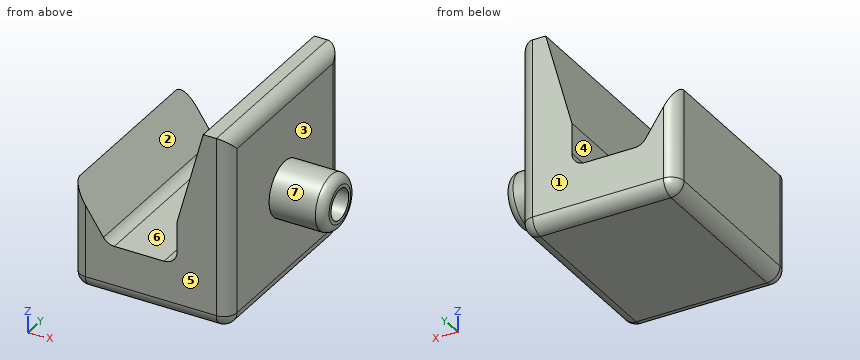
```python
from build123d import *

# Parameters (mm, degrees)
F1_DEPTH      = 11
F1_DEPTH_BACK = 11
F2_R          = 3.135192
F2_R_2        = 1.742831
F3_DEPTH      = 6.3
F4_R          = 1.5
F5_R          = 1
F3_FACE_R     = 1.742831
F6_DEPTH      = 1.5


with BuildPart() as f1:
    # F0 (on Front) → F1 (new body, two sides)
    with BuildSketch(Plane.XZ) as f1_sk:
        Polygon((-3, -11), (3, -11), (3, -3.201166), (3, 0), (3, 3.152842), (3, 11), (0, 11), (-3, 0), (-3, -5), (-11.005839, -5), (-15, 1), (-15, -5), (-15, -11), align=None)
    extrude(amount=F1_DEPTH)
    extrude(f1_sk.sketch, amount=-F1_DEPTH_BACK)

    # F2 (on face) → F3 (join)
    with BuildSketch(Plane.YZ.offset(3)):
        Circle(F2_R)
        Circle(F2_R_2, mode=Mode.SUBTRACT)
    extrude(amount=F3_DEPTH)

    # F4
    f4_edges = [f1.edges().sort_by_distance(p)[0] for p in [
        (3, -11, 0),
        (-6, -11, -11),
        (-15, -11, -5),
        (3, 0, 11),
        (3, 11, 0),
        (3, 0, -11),
        (-15, 11, -5),
        (-15, 0, -11),
        (-6, 11, -11),
        (-3, 0, -5),
        (-11.005839, 0, -5),
    ]]
    fillet(f4_edges, radius=F4_R)

    # F5
    f5_edges = [f1.edges().sort_by_distance(p)[0] for p in [
        (9.3, -3.135192, 0),
    ]]
    fillet(f5_edges, radius=F5_R)

    # F3_face (on face) → F6 (join)
    with BuildSketch(Plane.YZ.offset(3)):
        Circle(F3_FACE_R)
    extrude(amount=-F6_DEPTH)


solid = f1.part
```
Read the model definition and answer for the solid it produces. Units are mm, in the model's axes. Face numbers are marked on the shaded views. A direction names the side the tool comes from. Give positions to 0.01 mm unless a question says otherwise; leave off trailing zeros. Write each loop counter-clockwise with the first axis right and the second up, starting at its lowest first coordinate (ties: lowest second). Pieces come first, ordered by that corner, then holes. Notation, with made-up numbers: (63, 73) -> (114, 73) arc R23 ccw to (114, 102) -> close; hole circle Ø2 at (1.25, 69.25). An arc over 180 degrees is marked (long way). Answer as a JSON object with one key per item and string values.
1) Section D-D on x = 6 is taken. Write down the section's boundary in (y, z).
Findings below:
{"outline": "circle Ø6.27 at (0, 0); hole circle Ø3.49 at (0, 0)"}
2) A tool of negligible diameter and unlimited length cuts with its end or side. For the marked faces 5, 6 and 7, from which of +Z, -Z, +X, -X, +Y, -Y can it reach the whole face along a straight path? Write none if from no direction.
Findings below:
{"face 5": "+Z, -Z, +X, -X, -Y", "face 6": "+Z, +Y, -Y", "face 7": "+X"}
3) Straight lines are drawn through the part: probe 1 along Z at (x, y) = (6.25, 0); probe 2 along Z at (x, y) = (-6.5, 3.25); probe 3 along X at (y, z) = (-7.5, -9.5). For each, find the intervals that lie inside material, in ascending order. Write a range as from..to.
Findings below:
{"probe 1": "z = -3.14..-1.74, 1.74..3.14", "probe 2": "z = -11..-5", "probe 3": "x = -15..3"}
4) Flat-ended cylindrical pins translate along their axes: pin 1 Ø4.5 at (x, y) = (-8, 2) entering from +Z; pin 2 Ø6 at (x, z) = (5, 8.5) entering from +Y; pin 3 Ø6 at (y, z) = (1.5, -7.5) entering from +X. Find the tip coordinate at first contact, or state that the pin passes through.
Findings below:
{"pin 1": "stops at z = -5", "pin 2": "stops at y = 10.91", "pin 3": "stops at x = 3"}
5) Section C-C on z = -5.75 is taken. Write down the section's boundary in (x, y), then the cut area to 3 significant figures.
Findings below:
{"outline": "(-15, -9.5) arc R1.5 ccw to (-13.5, -11) -> (1.5, -11) arc R1.5 ccw to (3, -9.5) -> (3, 9.5) arc R1.5 ccw to (1.5, 11) -> (-13.5, 11) arc R1.5 ccw to (-15, 9.5) -> close", "area": "394 mm^2"}
6) Section B-B on x = -7 is taken. Write down the section's boundary in (y, z).
Findings below:
{"outline": "(-11, -9.5) arc R1.5 ccw to (-9.5, -11) -> (9.5, -11) arc R1.5 ccw to (11, -9.5) -> (11, -5) -> (-11, -5) -> close"}
7) Section A-A on y = 0 is taken. Write down the section's boundary in (x, z).
Findings below:
{"outline": "(-15, -9.5) arc R1.5 ccw to (-13.5, -11) -> (1.5, -11) arc R1.5 ccw to (3, -9.5) -> (3, -3.14) -> (8.3, -3.14) arc R1 ccw to (9.3, -2.14) -> (9.3, -1.74) -> (3, -1.74) -> (3, 1.74) -> (9.3, 1.74) -> (9.3, 2.14) arc R1 ccw to (8.3, 3.14) -> (3, 3.14) -> (3, 9.5) arc R1.5 ccw to (1.5, 11) -> (0, 11) -> (-3, 0) -> (-3, -3.5) arc R1.5 cw to (-4.5, -5) -> (-10.2, -5) arc R1.5 cw to (-11.45, -4.33) -> (-15, 1) -> close"}
8) For a pull along X with two mould halves and no side action, classify the marked faces 1, 2, 3 and 4 as pulls with the +X half, pulls with the -X half, needs draft (parallel to the pull), parting line crosses it, or undercut.
Findings below:
{"face 1": "needs draft", "face 2": "undercut", "face 3": "pulls with the +X half", "face 4": "undercut"}
